The model under review builds one solid part; all positions refer to its coordinate system, in mm. A direction names the side the tool comes from. Round coordinates to 2 decimals unless told otherwise and drop trailing zeros. Write each loop counter-clockwise with the first axis right and the second up, starting at its lowest first coordinate (ties: lowest second). Pieces come first, ordered by that corner, then holes. Notation, with made-up numbers: (48, -40) - (75, -40) arc R27 cw to (75, -18) - close; hole circle Ø8 at (76.25, 6.25). An arc over 180 degrees is marked (long way). Write each question's results on one line, items separated by ' | '.
Autodesk Inventor part; units mm, degrees
ref_plane "YZ Plane" through (0, 0, 0) normal (1, 0, 0) x (0, 1, 0)
ref_plane "XZ Plane" through (0, 0, 0) normal (0, 1, 0) x (-1, 0, 0)
ref_plane "XY Plane" through (0, 0, 0) normal (0, 0, 1) x (1, 0, 0)
ref_plane "Work Plane1" through (0, -1.5, -1) normal (0, 0, 1) x (1, 0, 0)
sketch "Sketch1" plane through (0, -1.5, -1) normal (0, 0, 1) x (1, 0, 0)
  line L0 (-2.8412, 5.5) -> (-2.8412, 7.5)
  line L1 (-2.8412, 5.5) -> (-2.8412, 7.5)
  line L2 (-2.8412, 5.5) -> (-2.8412, 7.5)
  line L3 (-2.8412, 7.5) -> (0, 7.5)
  line L4 (-2.8412, 5.5) -> (0, 5.5)
  line L5 (0, 5.5) -> (0, 7.5)
  line L6 (0, 7.5) -> (-2.8412, 7.5)
  line L7 (-2.8412, 7.5) -> (-2.8412, 5.5)
  line L8 (-2.8412, 7.5) -> (-2.8412, 9)
  line L9 (-2.8412, 9) -> (-4.3412, 9)
  line L10 (0, 5.5) -> (0, 4)
  line L11 (0, 4) -> (1.5, 4)
  line L12 (1.5, 4) -> (-4.3412, 4)
  line L13 (-4.3412, 4) -> (-4.3412, 9)
  line L14 (-4.3412, 9) -> (1.5, 9)
  line L15 (1.5, 9) -> (1.5, 4)
  line L16 (-4.3412, 4) -> (-4.3412, -7)
  line L17 (-4.3412, -7) -> (-34.3412, -7)
  line L18 (-4.3412, 9) -> (-4.3412, 20)
  line L19 (-4.3412, 20) -> (-34.3412, 20)
  line L20 (-34.3412, 20) -> (-34.3412, -7)
  line L21 (-4.3412, -7) -> (-4.3412, -5)
  line L22 (-4.3412, -5) -> (-6.3412, -5)
  line L23 (-34.3412, 20) -> (-34.3412, 18)
  line L24 (-34.3412, 18) -> (-32.3412, 18)
  line L25 (-6.3412, -5) -> (-32.3412, -5)
  line L26 (-32.3412, -5) -> (-32.3412, 18)
  line L27 (-32.3412, 18) -> (-6.3412, 18)
  line L28 (-6.3412, 18) -> (-6.3412, -5)
  point P0 (0, 1.5)
  point P1 (-0.8412, 6.5)
  dimension "d0" = 1.5
  dimension "d1" = 1.5
  dimension "d2" = 1.5
  dimension "d3" = 1.5
  dimension "d4" = 11
  dimension "d5" = 30
  dimension "d6" = 11
  dimension "d7" = 2
  dimension "d8" = 2
  dimension "d9" = 2
  dimension "d10" = 2
extrude "Extrusion1" add sketch "Sketch1" along normal blind 2 contours L4 L10 L12 L13 L9 L8 L0 | L8 L14 L15 L11 L10 L5 L3 | L13 L16 L22 L28 L27 L24 L20 L19 L18 | L16 L17 L20 L24 L26 L25 L22
sketch "Sketch2" plane through (0, -1.5, 1) normal (0, 0, 1) x (1, 0, 0)
  line L0 (-34.3412, -7) -> (-4.3412, -7)
  line L1 (-4.3412, 20) -> (-34.3412, 20)
  line L2 (-6.3412, -5) -> (-19.3412, -5)
  line L3 (-6.3412, -5) -> (-32.3412, -5)
  line L4 (-19.3412, -5) -> (-22.3412, -5)
  line L5 (-6.3412, 18) -> (-19.3412, 18)
  line L6 (-32.3412, 18) -> (-6.3412, 18)
  line L7 (-19.3412, 18) -> (-22.3412, 18)
  line L8 (-22.3412, -5) -> (-24.3412, -5)
  line L9 (-24.3412, -5) -> (-24.3412, -7)
  line L10 (-24.3412, -7) -> (-22.3412, -7)
  line L11 (-22.3412, -7) -> (-22.3412, -5)
  line L12 (-22.3412, 18) -> (-24.3412, 18)
  line L13 (-24.3412, 18) -> (-24.3412, 20)
  line L14 (-24.3412, 20) -> (-22.3412, 20)
  line L15 (-22.3412, 20) -> (-22.3412, 18)
  line L16 (-19.3412, 18) -> (-17.3412, 18)
  line L17 (-17.3412, 18) -> (-17.3412, 20)
  line L18 (-17.3412, 20) -> (-19.3412, 20)
  line L19 (-19.3412, 20) -> (-19.3412, 18)
  line L20 (-19.3412, -5) -> (-17.3412, -5)
  line L21 (-17.3412, -5) -> (-17.3412, -7)
  line L22 (-17.3412, -7) -> (-19.3412, -7)
  line L23 (-19.3412, -7) -> (-19.3412, -5)
  point P0 (0, 1.5)
  dimension "d13" = 13
  dimension "d14" = 3
  dimension "d15" = 2
  dimension "d16" = 2
  dimension "d17" = 2
  dimension "d18" = 2
extrude "Extrusion2" add sketch "Sketch2" along normal blind 2 contours L9 L3 L11 L0 | L23 L2 L21 L0 | L17 L5 L19 L1 | L15 L6 L13 L1
sketch "Sketch3" plane through (0, -1.5, 1) normal (0, 0, 1) x (1, 0, 0)
  line L0 (-2.8412, 5.5) -> (-2.8412, 7.5)
  line L1 (-2.8412, 7.5) -> (0, 7.5)
  line L2 (0, 7.5) -> (0, 5.5)
  line L3 (0, 5.5) -> (-2.8412, 5.5)
  line L4 (-2.8412, 7.5) -> (-2.8412, 8.15)
  line L5 (-2.8412, 8.15) -> (-3.4912, 8.15)
  line L6 (-2.8412, 5.5) -> (0, 5.5)
  line L7 (0, 5.5) -> (0, 4.85)
  line L8 (0, 4.85) -> (0.65, 4.85)
  line L9 (0.65, 4.85) -> (-3.4912, 4.85)
  line L10 (-3.4912, 4.85) -> (-3.4912, 8.15)
  line L11 (-3.4912, 8.15) -> (0.65, 8.15)
  line L12 (0.65, 8.15) -> (0.65, 4.85)
  point P0 (0, 1.5)
  dimension "d21" = 0.65
  dimension "d22" = 0.65
  dimension "d23" = 0.65
  dimension "d24" = 0.65
extrude "Extrusion3" cut sketch "Sketch3" against normal up to next contours L3 L7 L9 L10 L5 L4 L0 | L4 L11 L12 L8 L7 L2 L1
equation "\"d6\" = d4"
equation "\"d21\" = d24"
equation "\"d22\" = d24"
equation "\"d23\" = d24"
properties part number "back_pack_side_3"
Q1. We need section D-D (y = 8.75). State the section outline as (x, z) points, plus the area to 3 significant figures.
Evaluation:
outline: (-34.34, -1) - (-32.34, -1) - (-32.34, 1) - (-34.34, 1) - close; (-6.34, -1) - (-4.34, -1) - (-4.34, 1) - (-6.34, 1) - close | area: 8.00 mm^2
Q2. We need section A-A (x = -7.5). State the section outline as (y, z) points.
Evaluation:
outline: (-8.5, -1) - (-6.5, -1) - (-6.5, 1) - (-8.5, 1) - close; (16.5, -1) - (18.5, -1) - (18.5, 1) - (16.5, 1) - close
Q3. The part is to be moulded in two halves that separate along Y. For faces 4 (the flat face through (-32.341, 5, 0)), 5 (the flat face through (-21, 18, 1)), 6 (the flat face through (-19, 18.5, 1)), say which applies: released by +Y, released by -Y, zero draft, split by the parting line, or undercut.
Evaluation:
face 4: undercut | face 5: zero draft | face 6: released by +Y
Q4. We need section C-C (y = 4.75). State the section outline as (x, z) points, plus the area to 3 significant figures.
Evaluation:
outline: (-34.34, -1) - (-32.34, -1) - (-32.34, 1) - (-34.34, 1) - close; (-6.34, -1) - (-3.49, -1) - (-3.49, 1) - (-6.34, 1) - close; (0.65, -1) - (1.5, -1) - (1.5, 1) - (0.65, 1) - close | area: 11.4 mm^2
Q5. Tool access review of faces 1 (the flat face through (-22.341, 18, 2)), 2 (the flat face through (-6, 6, 1)), 3 (the flat face through (-4.341, 13, 0)): name each direction out of +Z, -Z, +X, -X, +Y, -Y from which nothing blocks a thin tool from reaching the whole face with its end or side.
Evaluation:
face 1: +Z, +Y, -Y | face 2: +Z, +X, +Y, -Y | face 3: +Z, -Z, +X, +Y
Q6. We need section B-B (z = 1.95). State the section outline as (x, y) points.
Evaluation:
outline: (-24.34, -8.5) - (-22.34, -8.5) - (-22.34, -6.5) - (-24.34, -6.5) - close; (-24.34, 16.5) - (-22.34, 16.5) - (-22.34, 18.5) - (-24.34, 18.5) - close; (-19.34, -8.5) - (-17.34, -8.5) - (-17.34, -6.5) - (-19.34, -6.5) - close; (-19.34, 16.5) - (-17.34, 16.5) - (-17.34, 18.5) - (-19.34, 18.5) - close
Q7. Insertion check: P1, Ø5, axis at x = -6, y = 10, coming from the +Z side; P2, Ø1.6, axis at y = 17, z = 2.5, coming from the +X side; P3, Ø1, axis at y = 17.5, z = 2, coming from the -X side. Each pin has a flat end and moves straight along its axis. Give the tip position at first contact, or say it passes through.
Evaluation:
P1: stops at z = 1 | P2: stops at x = -17.34 | P3: stops at x = -24.34
Q8. For probe 1 along X at (y, z) = (5.25, 0); probe 2 along X at (y, z) = (9, 0.8); probe 3 along Y at (x, z) = (-19, 2.75), list the stretches that pass through material, from the lowest coordinate up.
Evaluation:
probe 1: x = -34.34 to -32.34, -6.34 to -3.49, 0.65 to 1.5 | probe 2: x = -34.34 to -32.34, -6.34 to -4.34 | probe 3: y = -8.5 to -6.5, 16.5 to 18.5
